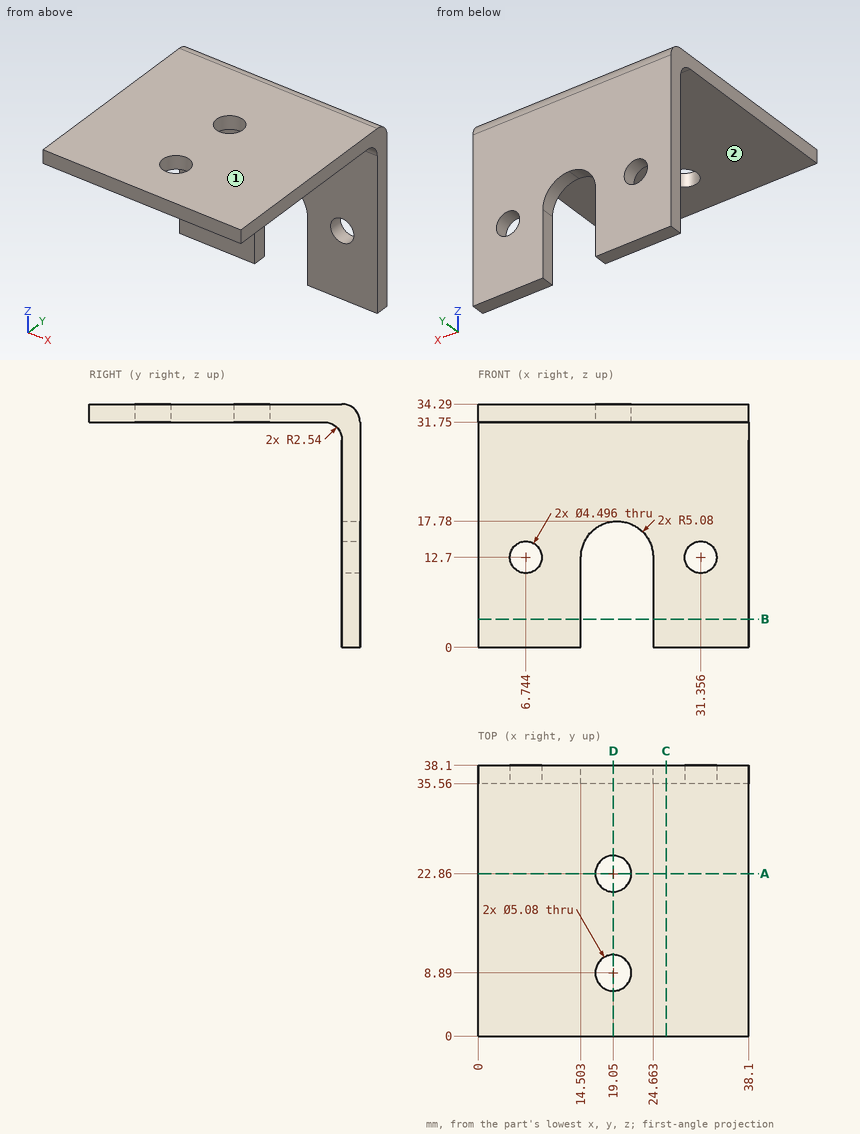
Design review of the part shown in the three views and the two pictorial views. Dimensions are in mm from the part's minimum x, y and z. A direction names the side the tool comes from. Give positions to 0.01 mm unless a question says otherwise; leave off trailing zeros. Loops run counter-clockwise (first coordinate to the right, second up) from the corner with the lowest first, then second, coordinate; pieces in that order, holes last. Notation, with made-up numbers: M 10,29.25 L 24,29.25 A16 cw 24,43.25 Z; hole C -27,74.25 d6. An arc over 180 degrees is marked long. Put each result on its own line as item: value. Start each with the question number.
(1) Add section C-C, the plane x = 26.5. Write out the cut boundary in (y, z).
(2) Add section B-B, the plane z = 4. Write out the cut boundary in (x, y).
(3) Machinability: for the marked faces 1 and 2, which of the approach directions +Z, -Z, +X, -X, +Y, -Y give a long, thin tool a straight path to every point of the face, cutting with its end or side? Answer none if there is none.
(4) Add section D-D, the plane x = 19.05. Write out the cut boundary in (y, z).
(5) Add section A-A, the plane y = 22.86. Write out the cut boundary in (x, z).
(6) Wall thickness on L1, parallel to X at y = 37.5, z = 12.7; L2, parallel to Y at x = 19, z = 32; L3, parallel to Y at x = 19.05, z = 33.5: over which ranges is each line inside the solid? List them lowest first.
(7) For pin 1 (5 mm diameter, centred on x = 31.36, z = 12.7, fed in from -Y), flat-tipped, find the tip position at first contact; note if it passes through.
Result:
1. outline: M 0,31.75 L 33.02,31.75 A2.54 cw 35.56,29.21 L 35.56,0 L 38.1,0 L 38.1,31.75 A2.54 ccw 35.56,34.29 L 0,34.29 Z
2. outline: M 0,35.56 L 14.5,35.56 L 14.5,38.1 L 0,38.1 Z; M 24.66,35.56 L 38.1,35.56 L 38.1,38.1 L 24.66,38.1 Z
3. face 1: +Z, +X, -X, +Y, -Y
3. face 2: -Z, +X, -X, -Y
4. outline: M 0,31.75 L 6.35,31.75 L 6.35,34.29 L 0,34.29 Z; M 11.43,31.75 L 20.32,31.75 L 20.32,34.29 L 11.43,34.29 Z; M 25.4,31.75 L 33.02,31.75 A2.54 cw 35.56,29.21 L 35.56,17.75 L 38.1,17.75 L 38.1,31.75 A2.54 ccw 35.56,34.29 L 25.4,34.29 Z
5. outline: M 0,31.75 L 16.51,31.75 L 16.51,34.29 L 0,34.29 Z; M 21.59,31.75 L 38.1,31.75 L 38.1,34.29 L 21.59,34.29 Z
6. L1: x = 0 to 4.5, 8.99 to 14.5, 24.66 to 29.11, 33.6 to 38.1
6. L2: y = 0 to 6.35, 11.43 to 20.32, 25.4 to 38.09
6. L3: y = 0 to 6.35, 11.43 to 20.32, 25.4 to 37.4
7. pin 1: stops at y = 35.56
